from build123d import *

# Parameters (mm, degrees)
SKETCH1_W           = 72
SKETCH1_H           = 57.2
BOSS_EXTRUDE1_DEPTH = 9.9
SKETCH2_R           = 1.9
BOSS_EXTRUDE2_DEPTH = 4
SKETCH4_W           = 72
SKETCH4_H           = 23
BOSS_EXTRUDE3_DEPTH = 3
SHELL1_START        = -26.6
SHELL1_OUTLINE_W    = 68
SHELL1_OUTLINE_H    = 15.8
SHELL1_DEPTH        = 59.2
SHELL1_START_2      = 30.6
SHELL1_2_OUTLINE_R  = 3.9
SHELL1_2_OUTLINE_W  = 68
SHELL1_2_OUTLINE_H  = 15.8
SHELL1_2_DEPTH      = 2


# Read off the part's stored shape, not the designer's step: Shell1
with BuildPart() as part:
    # Sketch1 → Boss-Extrude1 (new, symmetric)
    with BuildSketch(Plane(origin=(0, 0, 0), x_dir=(1, 0, 0), z_dir=(0, 1, 0))):
        Rectangle(SKETCH1_W, SKETCH1_H)
    extrude(amount=BOSS_EXTRUDE1_DEPTH, both=True)

    # Sketch2 → Boss-Extrude2 (add)
    with BuildSketch(Plane.XY.offset(28.6)):
        with BuildLine():
            Line((-39.1, 13), (39.1, 13))
            Line((39.1, 13), (46.276725004, 3.94394577))
            ThreePointArc((46.276725004, 3.94394577), (47.65, 0), (46.276725004, -3.94394577))
            Line((46.276725004, -3.94394577), (39.1, -13))
            Line((39.1, -13), (-39.1, -13))
            Line((-39.1, -13), (-46.276725004, -3.94394577))
            ThreePointArc((-46.276725004, -3.94394577), (-47.65, 0), (-46.276725004, 3.94394577))
            Line((-46.276725004, 3.94394577), (-39.1, 13))
        make_face()
        with Locations((-41.3, 0)):
            Circle(SKETCH2_R, mode=Mode.SUBTRACT)
        with Locations((41.3, 0)):
            Circle(SKETCH2_R, mode=Mode.SUBTRACT)
    extrude(amount=BOSS_EXTRUDE2_DEPTH)

    # Sketch4 → Boss-Extrude3 (add)
    with BuildSketch(Plane(origin=(0, 0, -28.6), x_dir=(-1, 0, 0), z_dir=(0, 0, -1))):
        with Locations((0, 1.6)):
            Rectangle(SKETCH4_W, SKETCH4_H)
    extrude(amount=-BOSS_EXTRUDE3_DEPTH)

    # Shell1 outline → Shell1 (cut)
    with BuildSketch(Plane.XY.offset(SHELL1_START)):
        Rectangle(SHELL1_OUTLINE_W, SHELL1_OUTLINE_H)
    extrude(amount=SHELL1_DEPTH, mode=Mode.SUBTRACT)

    # Shell1 2 outline → Shell1 2 (cut)
    with BuildSketch(Plane.XY.offset(SHELL1_START_2)):
        with BuildLine():
            Line((-38.133077283, 11), (-44.709252562, 2.701758126))
            ThreePointArc((-44.709252562, 2.701758126), (-45.65, 0), (-44.709252562, -2.701758126))
            Line((-44.709252562, -2.701758126), (-38.133077283, -11))
            Line((-38.133077283, -11), (38.133077283, -11))
            Line((38.133077283, -11), (44.709252562, -2.701758126))
            ThreePointArc((44.709252562, -2.701758126), (45.65, 0), (44.709252562, 2.701758126))
            Line((44.709252562, 2.701758126), (38.133077283, 11))
            Line((38.133077283, 11), (-38.133077283, 11))
        make_face()
        with Locations((-41.3, 0)):
            Circle(SHELL1_2_OUTLINE_R, mode=Mode.SUBTRACT)
        Rectangle(SHELL1_2_OUTLINE_W, SHELL1_2_OUTLINE_H, mode=Mode.SUBTRACT)
        with Locations((41.3, 0)):
            Circle(SHELL1_2_OUTLINE_R, mode=Mode.SUBTRACT)
    extrude(amount=SHELL1_2_DEPTH, mode=Mode.SUBTRACT)


solid = part.part
Could you check a few things on this model? Use its own coordinates, in mm. A direction names the side the tool comes from. Give positions to 0.01 mm unless a question says otherwise; leave off trailing zeros. Order: outer loops, then holes, each group sorted by start corner. A loop starts at its lowest first (then second) coordinate and runs counter-clockwise, first axis right, second up.
Item 1: If we section it at C-C, the plane x = 41: Write out the boundary of the cut face in (y, z).
Item 2: I'm going to push flat-ended pins straight in: pin 1 (16.5 mm diameter, centred on x = -10.5, z = 11.5, fed in from +Y); pin 2 (12 mm diameter, centred on x = 20.5, y = 2.5, fed in from +Z); pin 3 (4.5 mm diameter, centred on x = -15, y = -2.5, fed in from +Z). Where does each tip first touch, or does it pass through?
Item 3: If we section it at A-A, the plane z = 22: Write out the boundary of the cut face in (x, y).
Item 4: I need wall thicknesses on line 1 (X direction, y = -2.75, z = -3.5); line 2 (Y direction, x = -20, z = 6); line 3 (Y direction, x = 41.3, z = 30.9). Which ranges of each line are inside material? Lowest first, please.
Item 5: For faces 4 (the face through (1, 12, -25.6)), 5 (the face through (-37.58, 1.17, 31.59)), 6 (the face through (-36, 2, 0)), which set-ups out of +Z, -Z, +X, -X, +Y, -Y let a thin tool reach every point of the face, with its end or its side?
Item 6: If we section it at D-D, the plane x = -7: Write out the boundary of the cut face in (y, z).
Item 7: If we section it at B-B, the plane y = 0: Count the separate pieces of the cut face and the enclosed holes in it, plus the area to 3 significant figures.
Item 8: If we mould it in two halves opening along Z, with no side actions, what happens to faces 1 (the face through (42.638, 8.535, 30.572)), 2 (the face through (-1, 9.9, 1)), 3 (the face through (-1, 2, -28.6))? For each: pulls with the +Z half, pulls with the -Z half, needs draft (parallel to the pull), parting line crosses it, or undercut.
Values:
1. outline: (-10.6, 28.6) - (-1.88, 28.6) - (-1.88, 32.6) - (-3.89, 32.6) - (-3.89, 30.6) - (-7.38, 30.6) - (-7.38, 32.6) - (-10.6, 32.6) - close; (1.88, 28.6) - (10.6, 28.6) - (10.6, 32.6) - (7.38, 32.6) - (7.38, 30.6) - (3.89, 30.6) - (3.89, 32.6) - (1.88, 32.6) - close
2. pin 1: stops at y = 9.9
2. pin 2: stops at z = 30.6
2. pin 3: stops at z = -26.6
3. outline: (-36, -9.9) - (36, -9.9) - (36, 9.9) - (-36, 9.9) - close; hole (-34, -7.9) - (34, -7.9) - (34, 7.9) - (-34, 7.9) - close
4. line 1: x = -36 to -34, 34 to 36
4. line 2: y = -9.9 to -7.9, 7.9 to 9.9
4. line 3: y = -10.22 to -7, -3.9 to -1.9, 1.9 to 3.9, 7 to 10.22
5. face 4: +X, -X, +Y
5. face 5: +Z
5. face 6: -Z, -X, +Y, -Y
6. outline: (-13, 28.6) - (-9.9, 28.6) - (-9.9, -28.6) - (13.1, -28.6) - (13.1, -25.6) - (9.9, -25.6) - (9.9, 28.6) - (13, 28.6) - (13, 32.6) - (11, 32.6) - (11, 30.6) - (7.9, 30.6) - (7.9, -26.6) - (-7.9, -26.6) - (-7.9, 30.6) - (-11, 30.6) - (-11, 32.6) - (-13, 32.6) - close
7. separate pieces: 3
7. enclosed holes: 0
7. area: 428 mm2
8. face 1: needs draft
8. face 2: undercut
8. face 3: pulls with the -Z half
